from build123d import *

# Parameters (mm, degrees)
SKETCH_2_R          = 1.5
EXTRUDE_1_DEPTH     = 10
CUT_EXTRUDE_1_DEPTH = 1
CHAMFER_1_SIZE      = 0.5
FILLET_1_R          = 0.2


with BuildPart() as part:
    # 草图1 → 旋转2 (revolve)
    with BuildSketch(Plane.XY, mode=Mode.PRIVATE) as revolve_2_sk:
        Polygon((0, 1.9), (1.5, 1.9), (3, 0), (0, 0), align=None)
    revolve(revolve_2_sk.sketch.rotate(Axis((0, 3.310292653, 0), (0, -1, 0)), 90), axis=Axis((0, 3.310292653, 0), (0, -1, 0)))

    # 草图2 → 凸台-拉伸1 (add)
    with BuildSketch(Plane(origin=(0, 1.9, 0), x_dir=(1, 0, 0), z_dir=(0, 1, 0))):
        with Locations(Location((0, 0, 0), (0, 0, 270))):
            Circle(SKETCH_2_R)
    extrude(amount=EXTRUDE_1_DEPTH)

    # 草图3 → 切除-拉伸1 (cut)
    with BuildSketch(Plane.XZ):
        Polygon((0, 1.154700538), (-1, 0.577350269), (-1, -0.577350269), (0, -1.154700538), (1, -0.577350269), (1, 0.577350269), align=None)
    extrude(amount=-CUT_EXTRUDE_1_DEPTH, mode=Mode.SUBTRACT)

    # 倒角1
    chamfer_1_edges = [part.edges().sort_by_distance(p)[0] for p in [
        (0, 11.9, -1.5),
    ]]
    chamfer(chamfer_1_edges, length=CHAMFER_1_SIZE)

    # 圆角1
    fillet_1_edges = [part.edges().sort_by_distance(p)[0] for p in [
        (0, 0, -3),
        (0, 1.9, -1.5),
    ]]
    fillet(fillet_1_edges, radius=FILLET_1_R)


solid = part.part
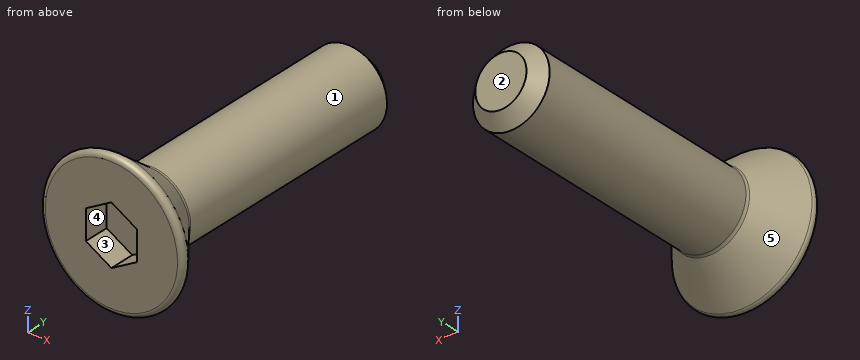
Check sheet for the modelled part. Datum: model origin and axes. Units: mm. Face numbers are marked on the shaded views. A direction names the side the tool comes from. Give positions to 0.01 mm unless a question says otherwise; leave off trailing zeros. Loops run counter-clockwise (first coordinate to the right, second up) from the corner with the lowest first, then second, coordinate; pieces in that order, holes last. Notation, with made-up numbers: M 34,78 L 57,78 A27 ccw 57,108 Z; hole C 29.25,87.5 d3. An arc over 180 degrees is marked long. Return JSON: item names as keys, results as strings. Group by question number.
1. Thickness scan on L1, parallel to Y at x = -0.05, z = 0.15; L2, parallel to Z at x = -0.35, y = 7.25; L3, parallel to Y at x = -1.65, z = 0. Record the ranges inside material, lowest first.
2. Go/stop test with flat-tipped pins: pin 1 (3 mm diameter, centred on y = 9, z = 1, fed in from -X); pin 2 (0.5 mm diameter, centred on y = 0.5, z = -0.5, fed in from -X); pin 3 (1.5 mm diameter, centred on y = 2.5, z = -1.5, fed in from -X). Record where each tip stops, or that it passes through.
3. Tool access check on the marked faces 4 and 5. Record the directions out of +Z, -Z, +X, -X, +Y, -Y that give a thin tool (end or side, any length) a straight path to the whole face; none if there is none.
4. Cross-section at A-A on y = 11. Record the boundary of the cut face in (x, z).
5. Mould release check, pull along X, two halves, no side actions. Record for the marked faces 1, 2 and 3: released by +X, released by -X, zero draft, split by the parting line, or undercut.
Return value:
{
 "1": {"L1": "1 to 11.9", "L2": "-1.46 to 1.46", "L3": "0 to 1.71"},
 "2": {"pin 1": "x = -1.5", "pin 2": "x = -2.75", "pin 3": "x = -1.3"},
 "3": {"face 4": "-Y", "face 5": "+Y"},
 "4": {"outline": "C 0,0 d3"},
 "5": {"face 1": "split by the parting line", "face 2": "zero draft", "face 3": "undercut"}
}
